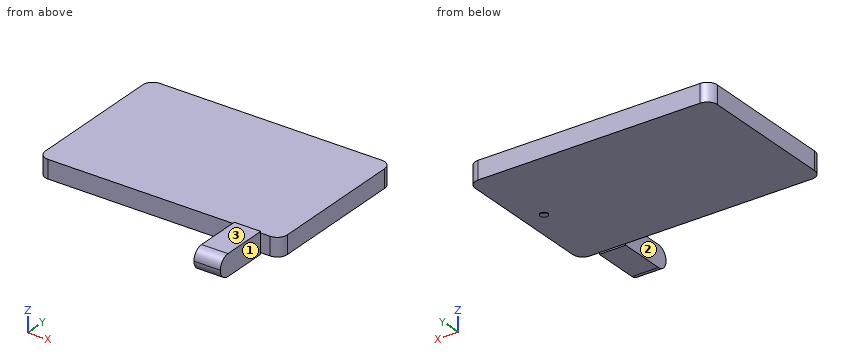
Autodesk Fusion 360 part; units mm, degrees
sketch "Sketch1" plane through (0, 0, 0) normal (0, 0, 1) x (1, 0, 0)
  line L0 (48.15, 31.15) -> (-48.15, 31.15)
  line L1 (-48.15, 31.15) -> (-48.15, -31.15)
  line L2 (-48.15, -31.15) -> (48.15, -31.15)
  line L3 (48.15, -31.15) -> (48.15, 31.15)
  line L4 (48.15, 31.15) -> (-48.15, -31.15) construction
  line L5 (-48.15, 31.15) -> (48.15, -31.15) construction
  line L6 (0, 0) -> (48.15, 0) construction
  circle A0 centre (40.15, 0) radius 1.5
  dimension "d1" = 96.3
  dimension "d2" = 62.3
  dimension "d10" = 3
  dimension "d11" = 8
extrude "Extrude1" add sketch "Sketch1" along normal blind 7.3 contours L0 L1 L2 L3 | A0
fillet "Fillet1" radius 4 4 edges at (-48.15, -31.15, 3.65) (48.15, -31.15, 3.65) (48.15, 31.15, 3.65) (-48.15, 31.15, 3.65)
extrude "Extrude2" add sketch "Sketch1" against normal blind 0.2 contours A0
sketch "Sketch3" plane through (0, -31.15, 0) normal (0, -1, 0) x (1, 0, 0)
  line L0 (44.15, 0) -> (44.15, 7.3)
  line L1 (44.15, 7.3) -> (-44.15, 7.3)
  line L2 (-44.15, 7.3) -> (-44.15, 0)
  line L3 (-44.15, 0) -> (44.15, 0)
  line L4 (48.15, 0) -> (48.15, 7.3) construction
  line L5 (48.15, 3.65) -> (35.15, 3.65) construction
  line L6 (40.4, -0.6) -> (29.9, -0.6)
  line L7 (29.9, -0.6) -> (29.9, 7.9)
  line L8 (29.9, 7.9) -> (40.4, 7.9)
  line L9 (40.4, 7.9) -> (40.4, -0.6)
  line L10 (40.4, -0.6) -> (29.9, 7.9) construction
  line L11 (29.9, -0.6) -> (40.4, 7.9) construction
  point P0 (35.15, 3.65)
  dimension "d16" = 13
  dimension "d17" = 10.5
  dimension "d18" = 8.5
extrude "Extrude3" add sketch "Sketch3" along normal blind 22.5 contours L3 L6 L7 L9 | L1 L3 L7 L9 | L1 L7 L8 L9
fillet "Fillet2" radius 4.25 2 edges at (35.15, -53.65, -0.6) (35.15, -53.65, 7.9)
equation "d1 = powerBankLength"
equation "d2 = powerBankWidth"
equation "clearanceStationary = 0.125 mm"
equation "clearanceMoving = 2 * clearanceStationary"
equation "powerBankWidth = 62.3 mm"
equation "powerBankLength = 96.3 mm"
equation "powerBankHeight = 7.3 mm"
equation "d8 = powerBankHeight"
equation "d17 = usbPlugWidth"
equation "d18 = usbPlugHeight"
equation "usbPlugWidth = 10.5 mm"
equation "usbPlugHeight = 8.5 mm"
equation "usbPlugLength = 22.5 mm"
equation "d22 = usbPlugLength"
equation "d25 = usbPlugHeight / 2"
Source: CAD feature listing. Evaluate the final solid. Frame: model axes, mm. Face numbers are marked on the shaded views. A direction names the side the tool comes from. Round coordinates to 2 decimals unless told otherwise and drop trailing zeros. Write each loop counter-clockwise with the first axis right and the second up, starting at its lowest first coordinate (ties: lowest second). Pieces come first, ordered by that corner, then holes. Notation, with made-up numbers: (71, 59) - (81, 59) arc R31 ccw to (81, 86) - close; hole circle Ø5 at (84, 43.5). An arc over 180 degrees is marked (long way). Use CSV: the item, a comma, the result in double quotes. Start each with the question number.
(1) Set-up query: the marked faces 1, 2 and 3. Return all of +Z, -Z, +X, -X, +Y, -Y with unobstructed straight access to the full face (end or side cutting, diameter ignored); none if empty.
(2) Cut plane D-D, the plane x = -21. Return loops of the section in (y, z).
(3) Material intervals for probe 1 along X at (y, z) = (-33, 6); probe 2 along Y at (x, z) = (18.5, 1.5); probe 3 along Z at (x, y) = (-15, 16), sorted ascending. Write a range as [from, to].
(4) Cut plane A-A, the plane y = 0. Return loops of the section in (x, z).
(5) First-contact query: pin 1 Ø1.5 at (x, y) = (-14.5, 6) entering from +Z; pin 2 Ø2 at (x, z) = (-9.5, 1.5) entering from -Y; pin 3 Ø1.5 at (x, y) = (40.5, 0) entering from -Z. Flat tips, straight axial feed; report the tip coordinate or a pass-through.
(6) Cut plane C-C, the plane y = -47.5. Return loops of the section in (x, z), and give its area (4 significant figures).
Geometry says:
1,face 1,"+Z, -Z, +X, -Y"
1,face 2,"+Z, -Z, -X, -Y"
1,face 3,"+Z, +X, -X, +Y, -Y"
2,outline,"(-31.15, 0) - (31.15, 0) - (31.15, 7.3) - (-31.15, 7.3) - close"
3,probe 1,"[29.9, 40.4]"
3,probe 2,"[-31.15, 31.15]"
3,probe 3,"[0, 7.3]"
4,outline,"(-48.15, 0) - (38.65, 0) - (38.65, -0.2) - (41.65, -0.2) - (41.65, 0) - (48.15, 0) - (48.15, 7.3) - (-48.15, 7.3) - close"
5,pin 1,"z = 7.3"
5,pin 2,"y = -31.15"
5,pin 3,"z = -0.2"
6,outline,"(29.9, -0.6) - (40.4, -0.6) - (40.4, 7.9) - (29.9, 7.9) - close"
6,area,"89.25 mm²"
